Verification items for this drawing (mm, ordinates from the low corner). A direction names the side the tool comes from. Round coordinates to 2 decimals unless told otherwise and drop trailing zeros. Write each loop counter-clockwise with the first axis right and the second up, starting at its lowest first coordinate (ties: lowest second). Pieces come first, ordered by that corner, then holes.
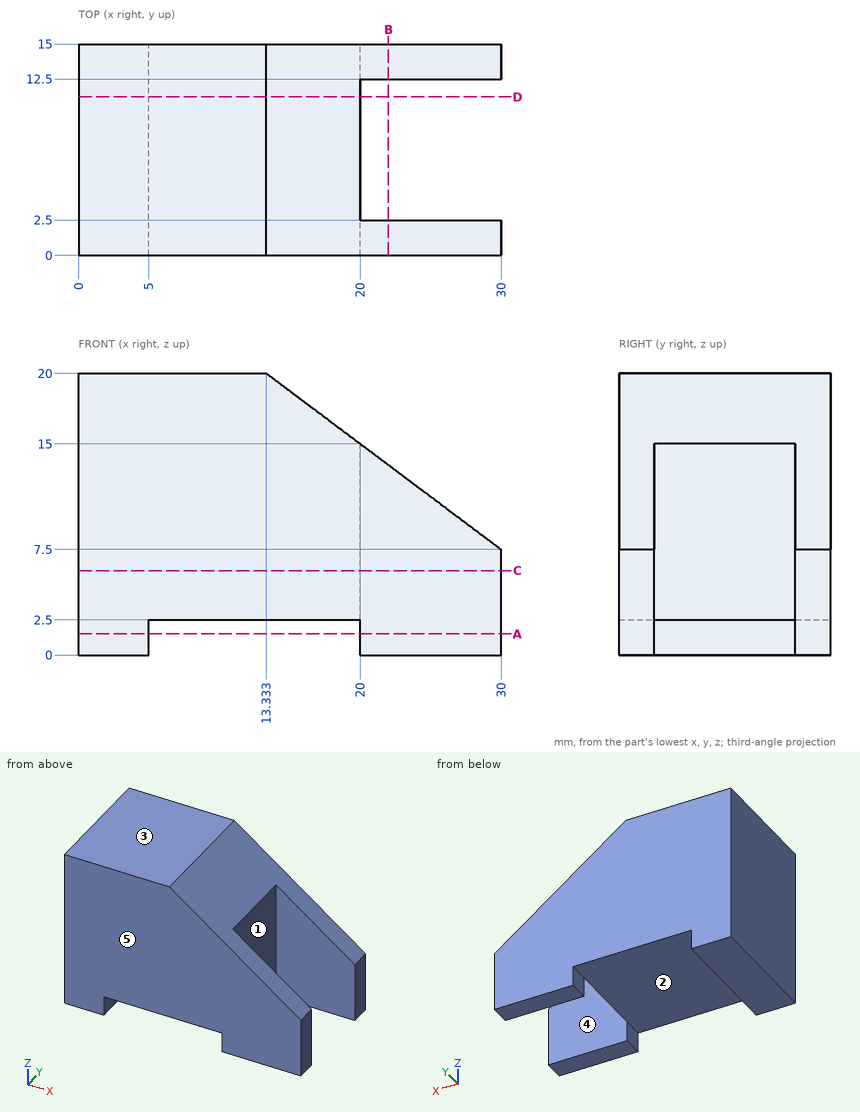
1. Section check B-B (x = 22). Record the cut outline in (y, z).
2. Release check for a two-part mould opening along X. For the marked faces 1, 2 and 3 record: +X half, -X half, draft (parallel to the pull), parting line (faces both ways), or undercut.
3. Section check A-A (z = 1.5). Record the cut outline in (x, y), plus the area to 3 significant figures.
4. Depth check by flat-ended pin: pin 1 Ø1.5 at (x, y) = (22.5, 13.5) entering from +Z; pin 2 Ø1.2 at (y, z) = (5.5, 1.5) entering from +X. Enter the tip coordinate at first touch or a pass-through.
5. Scan lines: line 1 along Y through (x, z) = (27.5, 4.5); line 2 along X through (y, z) = (6.75, 5.75); line 3 along X through (y, z) = (6.5, 1.75). Record each from-to range of solid material in increasing order.
6. Section check D-D (y = 11.25). Record the cut outline in (x, z), plus the area to 3 significant figures.
7. Access from +Z, -Z, +X, -X, +Y, -Y to the whole of each face (thin tool, end or side, straight path). Record for the marked faces 4 and 5.
8. Section check C-C (z = 6). Record the cut outline in (x, y), plus the area to 3 significant figures.
Results below:
1. outline: (0, 0) - (2.5, 0) - (2.5, 13.5) - (0, 13.5) - close; (12.5, 0) - (15, 0) - (15, 13.5) - (12.5, 13.5) - close
2. face 1: +X half
2. face 2: undercut
2. face 3: draft
3. outline: (0, 0) - (5, 0) - (5, 15) - (0, 15) - close; (20, 0) - (30, 0) - (30, 2.5) - (20, 2.5) - close; (20, 12.5) - (30, 12.5) - (30, 15) - (20, 15) - close
3. area: 125 mm2
4. pin 1: stops at z = 13.69
4. pin 2: stops at x = 5
5. line 1: y = 0 to 2.5, 12.5 to 15
5. line 2: x = 0 to 20
5. line 3: x = 0 to 5
6. outline: (0, 0) - (5, 0) - (5, 2.5) - (20, 2.5) - (20, 15) - (13.33, 20) - (0, 20) - close
6. area: 346 mm2
7. face 4: +Z, -Z, +X
7. face 5: +Z, -Z, +X, -X, -Y
8. outline: (0, 0) - (30, 0) - (30, 2.5) - (20, 2.5) - (20, 12.5) - (30, 12.5) - (30, 15) - (0, 15) - close
8. area: 350 mm2
